For this review, take the finished solid that the model builds, in its own axes (mm). Face numbers are marked on the shaded views. A direction names the side the tool comes from. Round coordinates to 2 decimals unless told otherwise and drop trailing zeros. Order: outer loops, then holes, each group sorted by start corner. A loop starts at its lowest first (then second) coordinate and runs counter-clockwise, first axis right, second up. Notation, with made-up numbers: (25, 9) -> (54, 9) arc R25 ccw to (54, 21) -> close; hole circle Ø7 at (-24, -30). An arc over 180 degrees is marked (long way). Answer in a Markdown table with one row per item.
```python
from build123d import *

# Parameters (mm, degrees)
F0_R      = 8
F1_DEPTH  = 5
F2_R      = 4
F3_DEPTH  = 6
F4_R      = 1.2
F5_DEPTH  = 9
F6_R      = 5
F7_DEPTH  = 2
F8_R      = 7.5
F8_R_2    = 6.75
F9_DEPTH  = 0.5
F10_SIZE  = 0.2
F11_R     = 0.2
F13_R     = 1.25
F14_DEPTH = 4.5
F15_R     = 8
F15_R_2   = 7
F16_DEPTH = 10
F17_R     = 7
F17_R_2   = 5.75
F18_DEPTH = 0.5


with BuildPart() as f1:
    # F0 (on Top) → F1 (new body)
    with BuildSketch(Plane.XY):
        Circle(F0_R)
    extrude(amount=F1_DEPTH)

    # F2 (on face) → F3 (join)
    with BuildSketch(Plane(origin=(0, 0, 0), x_dir=(1, 0, 0), z_dir=(0, 0, -1))):
        Circle(F2_R)
    extrude(amount=F3_DEPTH)

    # F4 (on face) → F5 (cut)
    with BuildSketch(Plane(origin=(0, 0, -6), x_dir=(1, 0, 0), z_dir=(0, 0, -1))):
        Circle(F4_R)
    extrude(amount=-F5_DEPTH, mode=Mode.SUBTRACT)

    # F6 (on face) → F7 (cut)
    with BuildSketch(Plane.XY.offset(5)):
        Circle(F6_R)
    extrude(amount=-F7_DEPTH, mode=Mode.SUBTRACT)

    # F8 (on face) → F9 (cut)
    with BuildSketch(Plane.XY.offset(5)):
        Circle(F8_R)
        Circle(F8_R_2, mode=Mode.SUBTRACT)
    extrude(amount=-F9_DEPTH, mode=Mode.SUBTRACT)

    # F10
    f10_edges = [f1.edges().sort_by_distance(p)[0] for p in [
        (-6.75, 0, 5),
    ]]
    chamfer(f10_edges, length=F10_SIZE)

    # F11
    f11_edges = [f1.edges().sort_by_distance(p)[0] for p in [
        (-6.75, 0, 4.8),
        (-1.2, 0, 3),
        (-1.2, 0, -6),
    ]]
    fillet(f11_edges, radius=F11_R)

    # F13 (on Right) → F14 (cut)
    with BuildSketch(Plane.YZ):
        with Locations((0, -3.5)):
            Circle(F13_R)
    extrude(amount=-F14_DEPTH, mode=Mode.SUBTRACT)

    # F15 (on face) → F16 (cut)
    with BuildSketch(Plane.XY.offset(5)):
        Circle(F15_R)
        Circle(F15_R_2, mode=Mode.SUBTRACT)
    extrude(amount=-F16_DEPTH, mode=Mode.SUBTRACT)

    # F17 (on face) → F18 (cut)
    with BuildSketch(Plane.XY.offset(5)):
        Circle(F17_R)
        Circle(F17_R_2, mode=Mode.SUBTRACT)
    extrude(amount=-F18_DEPTH, mode=Mode.SUBTRACT)


solid = f1.part
```
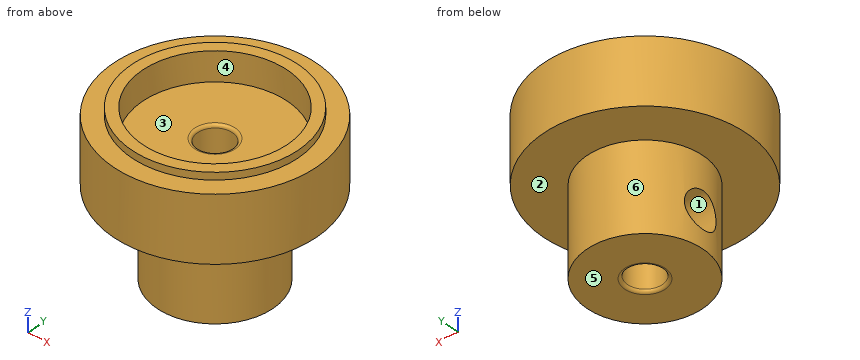
Q1. Clearance check with flat-ended pins moving along their axes: pin 1 Ø5 at (y, z) = (-3.5, -3) entering from +X; pin 2 Ø5 at (x, z) = (2.5, -4) entering from -Y; pin 3 Ø2 at (y, z) = (5.5, 1) entering from -X. State where each tip first meets the part, or that it passes through.
Answer key:
| item | result |
|---|---|
| pin 1 | stops at x = 3.87 |
| pin 2 | stops at y = -4 |
| pin 3 | stops at x = -5.36 |
Q2. The part is to be moulded in two halves that separate along Y. For the marked faces 4, 5 and 6, say which applies: +Y half, -Y half, draft (parallel to the pull), parting line (faces both ways), or undercut.
Answer key:
| item | result |
|---|---|
| face 4 | undercut |
| face 5 | draft |
| face 6 | parting line |
Q3. Tool access review of the marked faces 1, 2 and 3: name each direction out of +Z, -Z, +X, -X, +Y, -Y from which nothing blocks a thin tool from reaching the whole face with its end or side.
Answer key:
| item | result |
|---|---|
| face 1 | -X |
| face 2 | -Z |
| face 3 | +Z |
Q4. Take a section at C-C, the plane z = 2.25. Write out the cut boundary in (x, y), then the cut area to 3 significant figures.
Answer key:
| item | result |
|---|---|
| outline | circle Ø14 at (0, 0); hole circle Ø2.4 at (0, 0) |
| area | 149 mm^2 |
Q5. Take a section at D-D, the plane y = 3.5. Write out the cut boundary in (x, z).
Answer key:
| item | result |
|---|---|
| outline | (-6.06, 0) -> (-1.94, 0) -> (-1.94, -6) -> (1.94, -6) -> (1.94, 0) -> (6.06, 0) -> (6.06, 4.5) -> (4.56, 4.5) -> (4.56, 5) -> (3.57, 5) -> (3.57, 3) -> (-3.57, 3) -> (-3.57, 5) -> (-4.56, 5) -> (-4.56, 4.5) -> (-6.06, 4.5) -> close |
Q6. Take a section at B-B, the plane x = -2.25. Write out the cut boundary in (y, z).
Answer key:
| item | result |
|---|---|
| outline | (-6.63, 0) -> (-3.31, 0) -> (-3.31, -6) -> (3.31, -6) -> (3.31, 0) -> (6.63, 0) -> (6.63, 4.5) -> (5.29, 4.5) -> (5.29, 5) -> (4.47, 5) -> (4.47, 3) -> (-4.47, 3) -> (-4.47, 5) -> (-5.29, 5) -> (-5.29, 4.5) -> (-6.63, 4.5) -> close; hole circle Ø2.5 at (0, -3.5) |
Q7. To check wall thickness, follow probe 1 along Y at (x, z) = (0, 3.65); probe 2 along X at (y, z) = (0, -1.25); probe 3 along Z at (x, y) = (4.5, -2.25). State the ranges of each line that lie inside material, in increasing order.
Answer key:
| item | result |
|---|---|
| probe 1 | y = -7 to -5, 5 to 7 |
| probe 2 | x = -4 to -1.2, 1.2 to 4 |
| probe 3 | z = 0 to 5 |
Q8. Take a section at A-A, the plane y = 0. Write out the cut boundary in (x, z).
Answer key:
| item | result |
|---|---|
| outline | (-7, 0) -> (-4, 0) -> (-4, -2.25) -> (-1.2, -2.25) -> (-1.2, 2.8) arc R0.2 ccw to (-1.4, 3) -> (-5, 3) -> (-5, 5) -> (-5.75, 5) -> (-5.75, 4.5) -> (-7, 4.5) -> close; (-4, -6) -> (-1.4, -6) arc R0.2 ccw to (-1.2, -5.8) -> (-1.2, -4.75) -> (-4, -4.75) -> close; (1.2, -5.8) arc R0.2 ccw to (1.4, -6) -> (4, -6) -> (4, 0) -> (7, 0) -> (7, 4.5) -> (5.75, 4.5) -> (5.75, 5) -> (5, 5) -> (5, 3) -> (1.4, 3) arc R0.2 ccw to (1.2, 2.8) -> close |
